Geometry: final body of the model. Coordinates: model frame, mm. Coordinates: 2 decimals unless noted, no trailing zeros. Loops run counter-clockwise (first coordinate to the right, second up) from the corner with the lowest first, then second, coordinate; pieces in that order, holes last. Notation, with made-up numbers: (-29, 61) - (12, 61) arc R21 ccw to (12, 99) - close; hole circle Ø1 at (-4.5, -29). An arc over 180 degrees is marked (long way). Put each result on its own line as item: value. Start each with the question number.
1) Section B-B on y = 61. Output: boundary loops of the cut face in (x, z).
2) Section C-C on z = 1.9. Output: boundary loops of the cut face in (x, y) (3 decimals).
3) Contact query for a flat-ended pin moving along its axis: pin 1 Ø1 at (x, y) = (64.5, 71) entering from -Z. Output: stop coordinate, or through.
4) Section A-A on x = 61.5. Output: boundary loops of the cut face in (y, z), and give its area (3 significant figures).
5) Material intervals for line 1 along Y through (x, z) = (33.5, 1.75); line 2 along X through (y, z) = (29.5, 2.65), sorted ascending. Write a range as from..to.
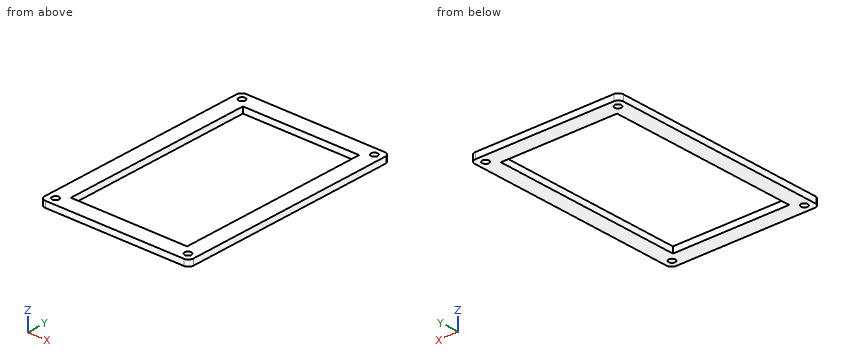
```python
from build123d import *

# Parameters (mm, degrees)
MODEL_R         = 1.625
MODEL_W         = 57.1502154
MODEL_H         = 95.249807
EXTRUDE_1_DEPTH = 3


with BuildPart() as part:
    # Model → 凸台-拉伸1 (new body)
    with BuildSketch(Plane.XY):
        with BuildLine():
            Line((8.022847613, 111.260961872), (2.522847613, 111.260961872))
            ThreePointArc((2.522847613, 111.260961872), (0.75508066, 110.528728825), (0.022847613, 108.760961872))
            Line((0.022847613, 108.760961872), (0.022847613, 8.011154872))
            Line((0.022847613, 8.011154872), (0.022847613, 2.511154872))
            ThreePointArc((0.022847613, 2.511154872), (0.75508066, 0.743387919), (2.522847613, 0.011154872))
            Line((2.522847613, 0.011154872), (65.173063013, 0.011154872))
            Line((65.173063013, 0.011154872), (70.673063013, 0.011154872))
            ThreePointArc((70.673063013, 0.011154872), (72.440829966, 0.743387919), (73.173063013, 2.511154872))
            Line((73.173063013, 2.511154872), (73.173063013, 8.011154872))
            Line((73.173063013, 8.011154872), (73.173063013, 108.760961872))
            ThreePointArc((73.173063013, 108.760961872), (72.440829966, 110.528728825), (70.673063013, 111.260961872))
            Line((70.673063013, 111.260961872), (8.022847613, 111.260961872))
        make_face()
        with Locations((69.173063013, 4.011154872)):
            Circle(MODEL_R, mode=Mode.SUBTRACT)
        with Locations((4.022847613, 4.011154872)):
            Circle(MODEL_R, mode=Mode.SUBTRACT)
        with Locations((4.022847613, 107.260961872)):
            Circle(MODEL_R, mode=Mode.SUBTRACT)
        with Locations((69.173063013, 107.260961872)):
            Circle(MODEL_R, mode=Mode.SUBTRACT)
        with Locations((36.597955313, 55.636058372)):
            Rectangle(MODEL_W, MODEL_H, mode=Mode.SUBTRACT)
    extrude(amount=EXTRUDE_1_DEPTH)


solid = part.part
```
Answer block:
1. outline: (0.02, 0) - (8.02, 0) - (8.02, 3) - (0.02, 3) - close; (65.17, 0) - (73.17, 0) - (73.17, 3) - (65.17, 3) - close
2. outline: (0.023, 2.511) arc R2.5 ccw to (2.523, 0.011) - (70.673, 0.011) arc R2.5 ccw to (73.173, 2.511) - (73.173, 108.761) arc R2.5 ccw to (70.673, 111.261) - (2.523, 111.261) arc R2.5 ccw to (0.023, 108.761) - close; hole circle Ø3.25 at (4.023, 4.011); hole circle Ø3.25 at (4.023, 107.261); hole (8.023, 8.011) - (65.173, 8.011) - (65.173, 103.261) - (8.023, 103.261) - close; hole circle Ø3.25 at (69.173, 4.011); hole circle Ø3.25 at (69.173, 107.261)
3. pin 1: passes through
4. outline: (0.01, 0) - (8.01, 0) - (8.01, 3) - (0.01, 3) - close; (103.26, 0) - (111.26, 0) - (111.26, 3) - (103.26, 3) - close
4. area: 48.0 mm²
5. line 1: y = 0.01..8.01, 103.26..111.26
5. line 2: x = 0.02..8.02, 65.17..73.17
